Can you work these out from the model? Positions are in its coordinate system, mm. A direction names the side the tool comes from. Give positions to 0.01 mm unless a question says otherwise; leave off trailing zeros. Order: outer loops, then holes, each group sorted by start corner. A loop starts at its lowest first (then second) coordinate and runs counter-clockwise, first axis right, second up. Notation, with made-up numbers: M 40.25,-18.75 L 49.25,-18.75 A28 ccw 49.25,20.25 Z; hole C 7.5,82.5 d10. An arc over 180 degrees is marked long. Write each question's results on one line, items separated by ' | '.
Autodesk Inventor part; units mm, degrees
ref_plane "YZ Plane" through (0, 0, 0) normal (1, 0, 0) x (0, 1, 0)
ref_plane "XZ Plane" through (0, 0, 0) normal (0, 1, 0) x (-1, 0, 0)
ref_plane "XY Plane" through (0, 0, 0) normal (0, 0, 1) x (1, 0, 0)
sketch "Sketch1" plane through (0, 0, 0) normal (0, 1, 0) x (-1, 0, 0)
  line L0 (-56.1975, 358.902) -> (56.1975, 358.902)
  line L1 (56.1975, 358.902) -> (56.1975, -358.902)
  line L2 (56.1975, -358.902) -> (-56.1975, -358.902)
  line L3 (-56.1975, -358.902) -> (-56.1975, 358.902)
  line L4 (-56.1975, 358.902) -> (56.1975, -358.902) construction
  line L5 (56.1975, 358.902) -> (-56.1975, -358.902) construction
  point P0 (0, 0)
  dimension "d0" = 112.395
  dimension "d1" = 717.804
extrude "Plate1" add sketch "Sketch1" along normal blind 3.048
sketch "Sketch2" plane through (56.1975, 0, 355.854) normal (0, 0, 1) x (1, 0, 0)
  line L0 (-112.395, 0) -> (0, 0)
  line L1 (0, 0) -> (0, 25.4)
  line L2 (0, 25.4) -> (-112.395, 25.4)
  line L3 (-112.395, 25.4) -> (-112.395, 0)
edge flange "Flange1" height 25.4 angle 90 thickness 3.048 bend radius 3.048 thickness toward (0, 0, 1) relief straight relief width 3.048 relief depth 1.524 corner gap 3.048 corner form 0 edges at (0, 3.048, 358.902) (0, 3.048, -358.902) wall of the first edge with corners at (-56.1975, 0, 355.854) (56.1975, 0, 355.854) (56.1975, 25.4, 355.854) (-56.1975, 25.4, 355.854)
bend "Bend1"
corner "Corner1"
equation "\"d5\" = BendReliefWidth"
equation "\"d6\" = BendReliefDepth"
equation "\"d7\" = MinimumRemnant"
equation "\"d8\" = BendRadius"
equation "\"d11\" = BendRadius"
equation "\"d12\" = CornerReliefSize"
equation "\"d13\" = GapSize"
equation "\"d14\" = JacobiRadiusSize"
equation "\"BendRadius\" = Thickness"
equation "\"BendReliefWidth\" = Thickness"
equation "\"BendReliefDepth\" = 0.5 * Thickness"
equation "\"CornerReliefSize\" = 4 * Thickness"
equation "\"MinimumRemnant\" = 2 * Thickness"
equation "\"TransitionRadius\" = BendRadius"
equation "\"JacobiRadiusSize\" = Thickness"
equation "\"GapSize\" = Thickness"
equation "\"d4\" = BendRadius"
properties part number "Side Gurad"
(1) Imagine slicing it at C-C, the plane z = 183. Write out the boundary of the cut face in (x, y).
Data:
outline: M -56.2,0 L 56.2,0 L 56.2,3.05 L -56.2,3.05 Z
(2) We'd pull the mould along Z, two halves only. Please class faces 1 (the face through (1, 16, 358.902)), 2 (the face through (-1, 16, -358.902)), 3 (the face through (56.198, 1, 2)), 4 (the face through (-1, 16, -355.854)): +Z half, -Z half, draft (parallel to the pull), parting line (faces both ways), or undercut.
Data:
face 1: +Z half | face 2: -Z half | face 3: draft | face 4: undercut
(3) Imagine slicing it at A-A, the plane y = 15.25. Write out the boundary of the cut face in (x, z), plus the area to 3 significant figures.
Data:
outline: M -56.2,-358.9 L 56.2,-358.9 L 56.2,-355.85 L -56.2,-355.85 Z; M -56.2,355.85 L 56.2,355.85 L 56.2,358.9 L -56.2,358.9 Z | area: 685 mm2
(4) I need wall thicknesses on L1, parallel to Z at x = -32.5, y = 12; L2, parallel to Y at x = 49.5, z = -193. Which ranges of each line are inside material? Lowest first, please. Write a range as from..to.
Data:
L1: z = -358.9..-355.85, 355.85..358.9 | L2: y = 0..3.05
(5) Will these pins go through, and if not, where does the flat tip stop? P1, Ø5, axis at x = -36.5, z = 97, coming from the +Y side; P2, Ø2, axis at x = 42, y = 3.5, coming from the -Z side.
Data:
P1: stops at y = 3.05 | P2: stops at z = -358.69
(6) For faces 5 (the face through (1, 3.048, 5)), 6 (the face through (-56.198, 1, 2)), which set-ups out of +Z, -Z, +X, -X, +Y, -Y let a thin tool reach every point of the face, with its end or its side?
Data:
face 5: +X, -X, +Y | face 6: +Z, -Z, -X, +Y, -Y
(7) Imagine slicing it at B-B, the plane x = -34.5. Write out the boundary of the cut face in (y, z).
Data:
outline: M 0,-352.81 A6.1 ccw 6.1,-358.9 L 25.4,-358.9 L 25.4,-355.85 L 6.1,-355.85 A3.05 cw 3.05,-352.81 L 3.05,352.81 A3.05 cw 6.1,355.85 L 25.4,355.85 L 25.4,358.9 L 6.1,358.9 A6.1 ccw 0,352.81 Z
